Geometry check sheet. Reference: the model listing, model coordinates, mm. A direction names the side the tool comes from. Round coordinates to 2 decimals unless told otherwise and drop trailing zeros. Write each loop counter-clockwise with the first axis right and the second up, starting at its lowest first coordinate (ties: lowest second). Pieces come first, ordered by that corner, then holes. Notation, with made-up numbers: M -18,-37.75 L 6,-37.75 A7 ccw 6,-24.75 Z; hole C -11.75,-29 d6. An arc over 180 degrees is marked long. Answer as CSV lines item,"result". Start each with the question number.
```python
from build123d import *

# Parameters (mm, degrees)
SKETCH1_W           = 250
SKETCH1_H           = 500
BOSS_EXTRUDE1_DEPTH = 110
SKETCH2_W           = 226
SKETCH2_H           = 474
CUT_EXTRUDE1_DEPTH  = 100
SKETCH3_W           = 226
SKETCH3_H           = 474
CUT_EXTRUDE2_DEPTH  = 7
SKETCH4_W           = 531.711239379
SKETCH4_H           = 96.104903681
CUT_EXTRUDE3_DEPTH  = 251
SKETCH5_W           = 125.68494841
SKETCH5_H           = 51.126080709
CUT_EXTRUDE4_DEPTH  = 15
FILLET1_R           = 8
CHAMFER1_SIZE       = 1
CHAMFER2_SIZE       = 1


with BuildPart() as part:
    # Sketch1 → Boss-Extrude1 (new body)
    with BuildSketch(Plane(origin=(0, 0, 0), x_dir=(1, 0, 0), z_dir=(0, 1, 0))):
        Rectangle(SKETCH1_W, SKETCH1_H)
    extrude(amount=BOSS_EXTRUDE1_DEPTH)

    # Sketch2 → Cut-Extrude1 (cut)
    with BuildSketch(Plane(origin=(0, 110, 0), x_dir=(1, 0, 0), z_dir=(0, 1, 0))):
        Rectangle(SKETCH2_W, SKETCH2_H)
    extrude(amount=-CUT_EXTRUDE1_DEPTH, mode=Mode.SUBTRACT)

    # Sketch3 → Cut-Extrude2 (cut)
    with BuildSketch(Plane.XZ):
        Rectangle(SKETCH3_W, SKETCH3_H)
    extrude(amount=-CUT_EXTRUDE2_DEPTH, mode=Mode.SUBTRACT)

    # Sketch4 → Cut-Extrude3 (cut, through all)
    with BuildSketch(Plane(origin=(125, 0, 0), x_dir=(0, 0, -1), z_dir=(1, 0, 0))):
        with Locations((27.855619689, 128.05245184)):
            Rectangle(SKETCH4_W, SKETCH4_H)
    extrude(amount=-CUT_EXTRUDE3_DEPTH, mode=Mode.SUBTRACT)

    # Sketch5 → Cut-Extrude4 (cut)
    with BuildSketch(Plane.XY.offset(250)):
        with Locations((0, 117.975615041)):
            Rectangle(SKETCH5_W, SKETCH5_H)
    extrude(amount=-CUT_EXTRUDE4_DEPTH, mode=Mode.SUBTRACT)

    # Fillet1
    fillet1_edges = [part.edges().sort_by_distance(p)[0] for p in [
        (62.842474205, 110, 244),
        (62.842474205, 92.412574686, 244),
        (-62.842474205, 110, 244),
        (-62.842474205, 92.412574686, 244),
    ]]
    fillet(fillet1_edges, radius=FILLET1_R)

    # Chamfer1
    chamfer1_edges = [part.edges().sort_by_distance(p)[0] for p in [
        (-97.921237103, 110, 250),
        (0, 0, 250),
        (125, 55, 250),
        (-125, 55, 250),
        (62.842474205, 101.206287343, 250),
        (0, 92.412574686, 250),
        (97.921237103, 110, 250),
        (-62.842474205, 101.206287343, 250),
        (-65.185619956, 107.656854249, 250),
        (65.185619956, 107.656854249, 250),
        (60.499328455, 94.755720436, 250),
        (-60.499328455, 94.755720436, 250),
    ]]
    chamfer(chamfer1_edges, length=CHAMFER1_SIZE)

    # Chamfer2
    chamfer2_edges = [part.edges().sort_by_distance(p)[0] for p in [
        (125, 110, 243.5),
        (125, 0, -0.5),
        (-125, 110, 243.5),
        (-125, 0, -0.5),
    ]]
    chamfer(chamfer2_edges, length=CHAMFER2_SIZE)


solid = part.part
```
1) Section check A-A, the plane y = 16.5. Record the cut outline in (x, z), plus the area to 3 significant figures.
2) Go/stop test with flat-tipped pins: pin 1 (12 mm diameter, centred on x = 22, z = 245.5, fed in from +Y); pin 2 (6 mm diameter, centred on x = 14.5, z = 130.5, fed in from -Y); pin 3 (6 mm diameter, centred on x = 28.5, z = 153.5, fed in from +Y). Record where each tip stops, or that it passes through.
3) Mould release check, pull along X, two halves, no side actions. Record for faces 6 (the flat face through (-98, 110, 243)), 7 (the conical face through (60.558, 94.57, 249.174)), 8 (the flat face through (125, 42, 3)): released by +X, released by -X, zero draft, split by the parting line, or undercut.
4) Section check B-B, the plane x = 15. Record the cut outline in (y, z).
5) Access from +Z, -Z, +X, -X, +Y, -Y to the whole of each face (thin tool, end or side, straight path). Record for faces 1 (the flat face through (-2, 7, 3)), 2 (the flat face through (2, 91, 238)), 3 (the conical face through (-60.685, 94.697, 249.174)), 4 (the flat face through (-1, 92.413, 244)), 5 (the flat face through (113, 45, 3)).
6) Section check C-C, the plane z = -35.5. Record the cut outline in (x, y), plus the area to 3 significant figures.
7) Scan lines: line 1 (X direction, y = 6.5, z = -1.5); line 2 (Z direction, x = 40.5, y = 74.5); line 3 (Z direction, x = 67, y = 91.5). Record each from-to range of solid material in increasing order. Write a range as from..to.
8) Section check D-D, the plane x = -89. Record the cut outline in (y, z), plus the area to 3 significant figures.
Results:
1,outline,"M -125,-250 L 125,-250 L 125,249 L 124,250 L -124,250 L -125,249 Z; hole M -113,-237 L 113,-237 L 113,237 L -113,237 Z"
1,area,"17,900 mm^2"
2,pin 1,"stops at y = 92.41"
2,pin 2,"stops at y = 7"
2,pin 3,"stops at y = 10"
3,face 6,"zero draft"
3,face 7,"undercut"
3,face 8,"released by +X"
4,outline,"M 0,-250 L 80,-250 L 80,-237 L 10,-237 L 10,237 L 80,237 L 80,238 L 92.41,238 L 92.41,249 L 91.41,250 L 1,250 L 0,249 L 0,237 L 7,237 L 7,-237 L 0,-237 Z"
5,face 1,"-Y"
5,face 2,"-Z, +X, -X, +Y"
5,face 3,"+Z, +Y"
5,face 4,"+Z, -Z, +Y"
5,face 5,"+Y"
6,outline,"M -125,1 L -124,0 L -113,0 L -113,7 L 113,7 L 113,0 L 124,0 L 125,1 L 125,80 L 113,80 L 113,10 L -113,10 L -113,80 L -125,80 Z"
6,area,"2,600 mm^2"
7,line 1,"x = -125..-113, 113..125"
7,line 2,"z = -250..-237, 237..250"
7,line 3,"z = 238..250"
8,outline,"M 0,-250 L 80,-250 L 80,-237 L 10,-237 L 10,237 L 80,237 L 80,238 L 110,238 L 110,249 L 109,250 L 1,250 L 0,249 L 0,237 L 7,237 L 7,-237 L 0,-237 Z"
8,area,"3,860 mm^2"
